from build123d import *

# Parameters (mm, degrees)
BOSS_EXTRUDE1_DEPTH = 45
M4_TAPPED_HOLE12_D  = 3.3
M4_TAPPED_HOLE13_D  = 3.3
SKETCH23_R          = 14.25
CUT_EXTRUDE5_DEPTH  = 3


with BuildPart() as part:
    # Sketch1 → Boss-Extrude1 (new body)
    with BuildSketch(Plane.XY):
        Polygon((0, 0), (53, 0), (53, 48), (50, 48), (50, 3), (0, 3), align=None)
    extrude(amount=BOSS_EXTRUDE1_DEPTH)

    # M4 Tapped Hole12 (through all)
    with Locations(Plane(origin=(0, 3, 0), x_dir=(1, 0, 0), z_dir=(0, 1, 0))):
        with Locations((38, -39), (12, -39), (12, -6), (38, -6)):
            Hole(M4_TAPPED_HOLE12_D / 2)

    # M4 Tapped Hole13 (through all)
    with Locations(Plane(origin=(53, 0, 0), x_dir=(0, 0, -1), z_dir=(1, 0, 0))):
        with Locations((-22.5, 44), (-5, 26.5), (-22.5, 9), (-40, 26.5)):
            Hole(M4_TAPPED_HOLE13_D / 2)

    # Sketch23 → Cut-Extrude5 (cut)
    with BuildSketch(Plane(origin=(53, 0, 0), x_dir=(0, 0, -1), z_dir=(1, 0, 0))):
        with Locations(Location((-22.5, 26.5, 0), (0, 0, 90))):
            Circle(SKETCH23_R)
    extrude(amount=-CUT_EXTRUDE5_DEPTH, mode=Mode.SUBTRACT)


solid = part.part
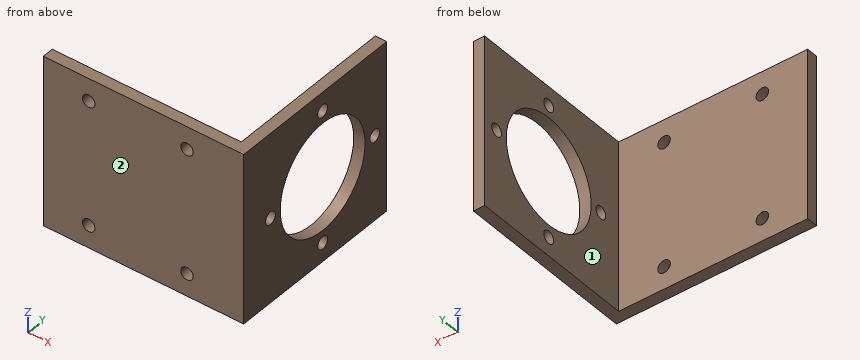
Here's how the part is built. I have some questions about the finished solid (model axes, mm). Face numbers are marked on the shaded views. A direction names the side the tool comes from. Round coordinates to 2 decimals unless told otherwise and drop trailing zeros. Loops run counter-clockwise (first coordinate to the right, second up) from the corner with the lowest first, then second, coordinate; pieces in that order, holes last. Notation, with made-up numbers: M 63,21 L 114,21 A21 ccw 114,31 Z; hole C 78,51 d7. An arc over 180 degrees is marked long. Write each question's results on one line, items separated by ' | '. Start each with the question number.
(1) I want a section at C-C (z = 22.5). Please give me the cut outline in (x, y), then the cut area to 3 significant figures.
(2) I want a section at D-D (y = 26.5). Please give me the cut outline in (x, z).
(3) On a 3-axis mill with a long thin cutter (end or side, diameter ignored), from which of +Z, -Z, +X, -X, +Y, -Y can I reach the whole of each face in a straight line? I mean the marked faces 1 and 2. Say none if no direction works.
(4) If I drill on probe 1 along X at (y, z) = (1, 39); probe 2 along X at (y, z) = (12.5, 14.5); probe 3 along Y at (x, z) = (17, 15.5), over which ranges is the centre line in solid material (lowest first)? Write a range as from..to.
(5) I want a section at B-B (y = 44). Please give me the cut outline in (x, z), then the cut area to 3 significant figures.
(6) Will these pins go through, and if not, where does the flat tip stop? P1, Ø13.5, axis at y = 20, z = 20, coming from the -X side; P2, Ø5.5, axis at x = 38, z = 6, coming from the +Y side; P3, Ø1.5, axis at y = 18, z = 33.5, coming from the -X side.
(7) I want a section at A-A (x = 38). Please give me the cut outline in (y, z), then the cut area to 3 significant figures.
Solved:
1) outline: M 0,0 L 53,0 L 53,7.35 L 50,7.35 L 50,3 L 0,3 Z; M 50,10.65 L 53,10.65 L 53,12.25 L 50,12.25 Z; M 50,40.75 L 53,40.75 L 53,42.35 L 50,42.35 Z; M 50,45.65 L 53,45.65 L 53,48 L 50,48 Z | area: 189 mm²
2) outline: M 50,0 L 53,0 L 53,3.35 L 50,3.35 Z; M 50,6.65 L 53,6.65 L 53,8.25 L 50,8.25 Z; M 50,36.75 L 53,36.75 L 53,38.35 L 50,38.35 Z; M 50,41.65 L 53,41.65 L 53,45 L 50,45 Z
3) face 1: +Z, -Z, -X, +Y | face 2: +Z, -Z, +X, -X, -Y
4) probe 1: x = 0..10.35, 13.65..36.35, 39.65..53 | probe 2: x = 50..53 | probe 3: y = 0..3
5) outline: M 50,0 L 53,0 L 53,20.85 L 50,20.85 Z; M 50,24.15 L 53,24.15 L 53,45 L 50,45 Z | area: 125 mm²
6) P1: passes through | P2: stops at y = 3 | P3: stops at x = 50
7) outline: M 0,0 L 3,0 L 3,4.35 L 0,4.35 Z; M 0,7.65 L 3,7.65 L 3,37.35 L 0,37.35 Z; M 0,40.65 L 3,40.65 L 3,45 L 0,45 Z | area: 115 mm²
